Read the model definition and answer for the solid it produces. Units are mm, in the model's axes. Face numbers are marked on the shaded views. Coordinates: 2 decimals unless noted, no trailing zeros. Write each loop counter-clockwise with the first axis right and the second up, starting at its lowest first coordinate (ties: lowest second). Pieces come first, ordered by that corner, then holes.
from build123d import *

# Parameters (mm, degrees)
SKETCH_1_R          = 2.1
SKETCH_1_R_2        = 2
SKETCH_1_W          = 8.5
SKETCH_1_H          = 2.2
EXTRUDE_1_DEPTH     = 8
CUT_EXTRUDE_START   = -8
SKETCH_2_R          = 2
CUT_EXTRUDE_2_DEPTH = 8
SKETCH_3_R          = 1.6
CUT_EXTRUDE_3_DEPTH = 10
SKETCH_4_R          = 3
CUT_EXTRUDE_4_DEPTH = 3


with BuildPart() as part:
    # 草图1 → 凸台-拉伸1 (new body)
    with BuildSketch(Plane(origin=(0, 0, 0), x_dir=(1, 0, 0), z_dir=(0, 1, 0))):
        with BuildLine():
            Line((0, 12.5), (50, 12.5))
            ThreePointArc((50, 12.5), (62.5, 0), (50, -12.5))
            Line((50, -12.5), (0, -12.5))
            ThreePointArc((0, -12.5), (-12.5, 0), (0, 12.5))
        make_face()
        with Locations(Location((0, 0, 0), (0, 0, 270))):
            Circle(SKETCH_1_R, mode=Mode.SUBTRACT)
        with Locations(Location((50, 0, 0), (0, 0, 270))):
            Circle(SKETCH_1_R_2, mode=Mode.SUBTRACT)
        with Locations((8.75, -2.1)):
            Rectangle(SKETCH_1_W, SKETCH_1_H, mode=Mode.SUBTRACT)
    extrude(amount=EXTRUDE_1_DEPTH)

    # 草图2 → 切除-拉伸2 (cut)
    with BuildSketch(Plane(origin=(0, 8, 0), x_dir=(1, 0, 0), z_dir=(0, 1, 0)).offset(CUT_EXTRUDE_START)):
        with Locations(Location((40, 0, 0), (0, 0, 270))):
            Circle(SKETCH_2_R)
        with Locations(Location((30, 0, 0), (0, 0, 270))):
            Circle(SKETCH_2_R)
        with Locations(Location((50, 0, 0), (0, 0, 270))):
            Circle(SKETCH_2_R)
    extrude(amount=CUT_EXTRUDE_2_DEPTH, mode=Mode.SUBTRACT)

    # 草图3 → 切除-拉伸3 (cut)
    with BuildSketch(Plane.XY.offset(12.5)):
        with Locations((9.051883486, 4.271448274)):
            Circle(SKETCH_3_R)
    extrude(amount=-CUT_EXTRUDE_3_DEPTH, mode=Mode.SUBTRACT)

    # 草图4 → 切除-拉伸4 (cut)
    with BuildSketch(Plane.XY.offset(12.5)):
        with Locations((9.051883486, 4.271448274)):
            Circle(SKETCH_4_R)
    extrude(amount=-CUT_EXTRUDE_4_DEPTH, mode=Mode.SUBTRACT)


solid = part.part
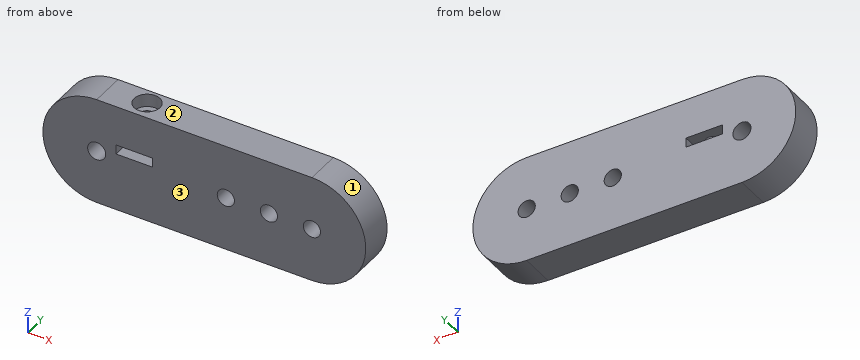
Item 1: The part is cut by section A-A (z = 0). Give the vertices of the cut face in (x, y), and give its area (3 significant figures).
Item 2: Find the intervals of material crossed by probe 1 along X at (y, z) = (2.25, 0); probe 2 along Z at (x, y) = (11, 5.75); probe 3 along Z at (x, y) = (41.5, 0.75), in increasing order.
Item 3: The part is cut by section B-B (x = 30). Give the vertices of the cut face in (y, z).
Item 4: The part is cut by section C-C (z = -4.75). Give the vertices of the cut face in (x, y), and give its area (3 significant figures).
Item 5: Determine the mould class of the marked faces 1, 2 and 3 for opening direction Z: +Z half, -Z half, draft (parallel to the pull), parting line (faces both ways), or undercut.
Item 6: Given pin 1 (3 mm diameter, centred on y = 2, z = -8.5, fed in from -X); pin 2 (1.1 mm diameter, centred on y = 2, z = 2, fed in from -X); pin 3 (4 mm diameter, centred on y = 3, z = -6, fed in from +X), each flat-ended and moving along its own axis, determine where each tip first touches the part or whether it passes through.
Answer:
1. outline: (-12.5, 0) - (-2.1, 0) - (-2.1, 8) - (-12.5, 8) - close; (2.1, 0) - (28, 0) - (28, 8) - (2.1, 8) - close; (32, 0) - (38, 0) - (38, 8) - (32, 8) - close; (42, 0) - (48, 0) - (48, 8) - (42, 8) - close; (52, 0) - (62.5, 0) - (62.5, 8) - (52, 8) - close
1. area: 470 mm2
2. probe 1: x = -12.5 to -2.1, 2.1 to 28, 32 to 38, 42 to 48, 52 to 62.5
2. probe 2: z = -12.5 to 1, 3.2 to 9.5
2. probe 3: z = -12.5 to -1.32, 1.32 to 12.5
3. outline: (0, -12.5) - (8, -12.5) - (8, -2) - (0, -2) - close; (0, 2) - (8, 2) - (8, 12.5) - (0, 12.5) - close
4. outline: (-11.56, 0) - (61.56, 0) - (61.56, 8) - (-11.56, 8) - close
4. area: 585 mm2
5. face 1: parting line
5. face 2: +Z half
5. face 3: draft
6. pin 1: stops at x = -10.36
6. pin 2: stops at x = -12.42
6. pin 3: stops at x = 61.84
